For this review, take the finished solid that the model builds, in its own axes (mm). Face numbers are marked on the shaded views. A direction names the side the tool comes from. Round coordinates to 2 decimals unless told otherwise and drop trailing zeros. Write each loop counter-clockwise with the first axis right and the second up, starting at its lowest first coordinate (ties: lowest second). Pieces come first, ordered by that corner, then holes. Notation, with made-up numbers: M -7.5,39.5 L 5.5,39.5 A32 cw 5.5,70.5 Z; hole C 7.5,-32.75 d10. An arc over 180 degrees is marked long. Answer in a Markdown table with one row per item.
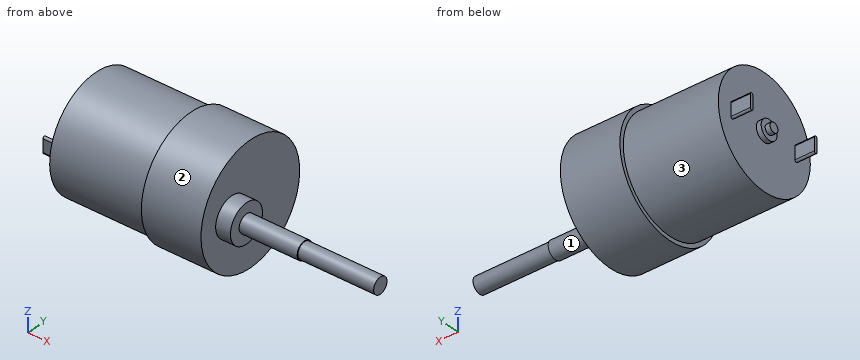
```python
from build123d import *

# Parameters (mm, degrees)
SKETCH1_R           = 17.25
BOSS_EXTRUDE1_DEPTH = 29.5
SKETCH2_R           = 18.5
BOSS_EXTRUDE2_DEPTH = 18.5
SKETCH3_R           = 3
BOSS_EXTRUDE3_DEPTH = 1.5
SKETCH4_R           = 1.5
BOSS_EXTRUDE4_DEPTH = 1.5
BOSS_EXTRUDE5_DEPTH = 6
SKETCH7_R           = 6
BOSS_EXTRUDE6_DEPTH = 4.6
SKETCH8_R           = 2.75
BOSS_EXTRUDE7_DEPTH = 18
SKETCH9_R           = 2.5
BOSS_EXTRUDE8_DEPTH = 23.54


with BuildPart() as part:
    # Sketch1 → Boss-Extrude1 (new body)
    with BuildSketch(Plane(origin=(0, 0, 0), x_dir=(0, 0, -1), z_dir=(1, 0, 0))):
        Circle(SKETCH1_R)
    extrude(amount=BOSS_EXTRUDE1_DEPTH)

    # Sketch2 → Boss-Extrude2 (add)
    with BuildSketch(Plane(origin=(29.5, 0, 0), x_dir=(0, 0, -1), z_dir=(1, 0, 0))):
        Circle(SKETCH2_R)
    extrude(amount=BOSS_EXTRUDE2_DEPTH)

    # Sketch3 → Boss-Extrude3 (add)
    with BuildSketch(Plane.ZY):
        Circle(SKETCH3_R)
    extrude(amount=BOSS_EXTRUDE3_DEPTH)

    # Sketch4 → Boss-Extrude4 (add)
    with BuildSketch(Plane.ZY.offset(1.5)):
        Circle(SKETCH4_R)
    extrude(amount=BOSS_EXTRUDE4_DEPTH)

    # Sketch5 → Boss-Extrude5 (add)
    with BuildSketch(Plane.ZY):
        with BuildLine():
            Line((-2, 12.5), (2, 12.5))
            ThreePointArc((2, 12.5), (2.5, 12), (2, 11.5))
            Line((2, 11.5), (-2, 11.5))
            ThreePointArc((-2, 11.5), (-2.5, 12), (-2, 12.5))
        make_face()
        with BuildLine():
            Line((-2, -12.5), (2, -12.5))
            ThreePointArc((2, -12.5), (2.5, -12), (2, -11.5))
            Line((2, -11.5), (-2, -11.5))
            ThreePointArc((-2, -11.5), (-2.5, -12), (-2, -12.5))
        make_face()
    extrude(amount=BOSS_EXTRUDE5_DEPTH)

    # Sketch7 → Boss-Extrude6 (add)
    with BuildSketch(Plane(origin=(48, 0, 0), x_dir=(0, 0, -1), z_dir=(1, 0, 0))):
        with Locations((0, -7)):
            Circle(SKETCH7_R)
    extrude(amount=BOSS_EXTRUDE6_DEPTH)

    # Sketch8 → Boss-Extrude7 (add)
    with BuildSketch(Plane(origin=(52.6, 0, 0), x_dir=(0, 0, -1), z_dir=(1, 0, 0))):
        with Locations((0, -7)):
            Circle(SKETCH8_R)
    extrude(amount=BOSS_EXTRUDE7_DEPTH)

    # Sketch9 → Boss-Extrude8 (add)
    with BuildSketch(Plane(origin=(70.6, 0, 0), x_dir=(0, 0, -1), z_dir=(1, 0, 0))):
        with Locations((0, -7)):
            Circle(SKETCH9_R)
    extrude(amount=BOSS_EXTRUDE8_DEPTH)


solid = part.part
```
Q1. Take a section at C-C (x = 43.5). State the section outline as (y, z) points, then the cut area to 3 significant figures.
Found:
| item | result |
|---|---|
| outline | C 0,0 d37 |
| area | 1,080 mm² |
Q2. Take a section at B-B (z = 10). State the section outline as (x, y) points.
Found:
| item | result |
|---|---|
| outline | M 0,-14.06 L 29.5,-14.06 L 29.5,-15.56 L 48,-15.56 L 48,15.56 L 29.5,15.56 L 29.5,14.06 L 0,14.06 Z |
Q3. Take a section at A-A (y = 0). State the section outline as (x, z) points, then the cut area to 3 significant figures.
Found:
| item | result |
|---|---|
| outline | M -3,-1.5 L -1.5,-1.5 L -1.5,-3 L 0,-3 L 0,-17.25 L 29.5,-17.25 L 29.5,-18.5 L 48,-18.5 L 48,18.5 L 29.5,18.5 L 29.5,17.25 L 0,17.25 L 0,3 L -1.5,3 L -1.5,1.5 L -3,1.5 Z |
| area | 1,720 mm² |
Q4. For probe 1 along X at (y, z) = (8.5, -12); probe 2 along X at (y, z) = (-11, -2); probe 3 along Z at (x, y) = (19.5, 14.5), list the stretches that pass through material, from the lowest coordinate up.
Found:
| item | result |
|---|---|
| probe 1 | 0 to 48 |
| probe 2 | 0 to 52.6 |
| probe 3 | -9.34 to 9.34 |
Q5. Insertion check: P1, Ø12, axis at y = 3.5, z = -13, coming from the +X side; P2, Ø2, axis at x = 5, y = -1.5, coming from the +Z side; P3, Ø4, axis at x = 59.5, y = -3, coming from the -Z side. Each pin has a flat end and moves straight along its axis. Give the tip position at first contact, or say it passes through.
Found:
| item | result |
|---|---|
| P1 | x = 48 |
| P2 | z = 17.24 |
| P3 | z = -1.89 |
Q6. Machinability: for the marked faces 1, 2 and 3, which of the approach directions +Z, -Z, +X, -X, +Y, -Y give a long, thin tool a straight path to every point of the face, cutting with its end or side? Answer none if there is none.
Found:
| item | result |
|---|---|
| face 1 | +X |
| face 2 | +X, -X |
| face 3 | -X |
Q7. Take a section at D-D (y = -7). State the section outline as (x, z) points, then the cut area to 3 significant figures.
Found:
| item | result |
|---|---|
| outline | M 0,-15.77 L 29.5,-15.77 L 29.5,-17.12 L 48,-17.12 L 48,-6 L 52.6,-6 L 52.6,-2.75 L 70.6,-2.75 L 70.6,-2.5 L 94.14,-2.5 L 94.14,2.5 L 70.6,2.5 L 70.6,2.75 L 52.6,2.75 L 52.6,6 L 48,6 L 48,17.12 L 29.5,17.12 L 29.5,15.77 L 0,15.77 Z |
| area | 1,840 mm² |
